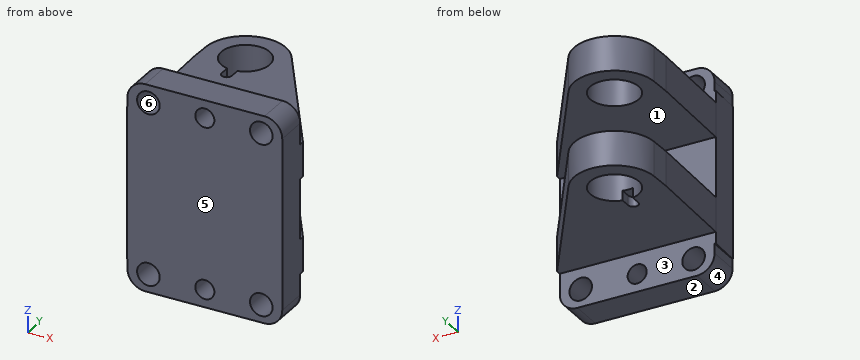
from build123d import *

# Parameters (mm, degrees)
SKETCH1_R                = 7
SKETCH1_R_2              = 5.9
BOSS_EXTRUDE1_DEPTH      = 20
BOSS_EXTRUDE2_DEPTH      = 47.15
BOSS_EXTRUDE2_DEPTH_BACK = 47.15
SKETCH3_R                = 15
BOSS_EXTRUDE3_DEPTH      = 21.4
SKETCH4_R                = 15
BOSS_EXTRUDE4_DEPTH      = 21.4
CUT_EXTRUDE1_DEPTH       = 6
CUT_EXTRUDE1_DEPTH_BACK  = 6
CUT_EXTRUDE2_DEPTH       = 6
CUT_EXTRUDE2_DEPTH_BACK  = 6


with BuildPart() as part:
    # Sketch1 → Boss-Extrude1 (new body)
    with BuildSketch(Plane(origin=(0, 0, 0), x_dir=(1, 0, 0), z_dir=(0, 1, 0))):
        with BuildLine():
            Line((-37, -64), (37, -64))
            ThreePointArc((37, -64), (44.778174593, -60.778174593), (48, -53))
            Line((48, -53), (48, 53))
            ThreePointArc((48, 53), (44.778174593, 60.778174593), (37, 64))
            Line((37, 64), (-37, 64))
            ThreePointArc((-37, 64), (-44.778174593, 60.778174593), (-48, 53))
            Line((-48, 53), (-48, -53))
            ThreePointArc((-48, -53), (-44.778174593, -60.778174593), (-37, -64))
        make_face()
        with Locations((35, 53)):
            Circle(SKETCH1_R, mode=Mode.SUBTRACT)
        with Locations((35, -53)):
            Circle(SKETCH1_R, mode=Mode.SUBTRACT)
        with Locations((0, 53)):
            Circle(SKETCH1_R_2, mode=Mode.SUBTRACT)
        with Locations((0, -53)):
            Circle(SKETCH1_R_2, mode=Mode.SUBTRACT)
        with Locations((-35, 53)):
            Circle(SKETCH1_R, mode=Mode.SUBTRACT)
        with Locations((-35, -53)):
            Circle(SKETCH1_R, mode=Mode.SUBTRACT)
    extrude(amount=BOSS_EXTRUDE1_DEPTH)

    # Sketch2 → Boss-Extrude2 (add, two sides)
    with BuildSketch(Plane.XY) as boss_extrude2_sk:
        Polygon((-48.744328002, 20), (-48.2, 0), (-43.2, 0), (-43.2, 20), align=None)
    extrude(amount=BOSS_EXTRUDE2_DEPTH)
    extrude(boss_extrude2_sk.sketch, amount=-BOSS_EXTRUDE2_DEPTH_BACK)

    # Sketch3 → Boss-Extrude3 (add)
    with BuildSketch(Plane.XY.offset(40)):
        with BuildLine():
            Line((-50.322839283, 77.998533118), (-48.2, 0))
            Line((-48.2, 0), (48, 0))
            Line((48, 0), (48, 22.55795714))
            ThreePointArc((48, 22.55795714), (47.938823082, 22.981971454), (47.760282483, 23.371399248))
            Line((47.760282483, 23.371399248), (-3.995291952, 103.55736847))
            ThreePointArc((-3.995291952, 103.55736847), (-31.752406245, 114.070833178), (-49.991433124, 90.654423708))
            Line((-49.991433124, 90.654423708), (-50.322839283, 77.998533118))
        make_face()
        with Locations((-25, 90)):
            Circle(SKETCH3_R, mode=Mode.SUBTRACT)
    extrude(amount=-BOSS_EXTRUDE3_DEPTH)

    # Sketch4 → Boss-Extrude4 (add)
    with BuildSketch(Plane.XY.offset(-40)):
        with BuildLine():
            Line((-50.322839283, 77.998533118), (-48.2, 0))
            Line((-48.2, 0), (48, 0))
            Line((48, 0), (48, 22.55795714))
            ThreePointArc((48, 22.55795714), (47.938823082, 22.981971454), (47.760282483, 23.371399248))
            Line((47.760282483, 23.371399248), (-3.995291952, 103.55736847))
            ThreePointArc((-3.995291952, 103.55736847), (-31.752406245, 114.070833178), (-49.991433124, 90.654423708))
            Line((-49.991433124, 90.654423708), (-50.322839283, 77.998533118))
        make_face()
        with Locations((-25, 90)):
            Circle(SKETCH4_R, mode=Mode.SUBTRACT)
    extrude(amount=BOSS_EXTRUDE4_DEPTH)

    # Sketch5 → Cut-Extrude1 (cut, two sides)
    with BuildSketch(Plane.XY.offset(40)) as cut_extrude1_sk:
        with BuildLine():
            Line((-21.85, 69.15), (-21.85, 90))
            Line((-21.85, 90), (-28.15, 90))
            Line((-28.15, 90), (-28.15, 69.15))
            ThreePointArc((-28.15, 69.15), (-25, 66), (-21.85, 69.15))
        make_face()
    extrude(amount=CUT_EXTRUDE1_DEPTH, mode=Mode.SUBTRACT)
    extrude(cut_extrude1_sk.sketch, amount=-CUT_EXTRUDE1_DEPTH_BACK, mode=Mode.SUBTRACT)

    # Sketch6 → Cut-Extrude2 (cut, two sides)
    with BuildSketch(Plane.XY.offset(-40)) as cut_extrude2_sk:
        with BuildLine():
            Line((-21.85, 69.15), (-21.85, 90))
            Line((-21.85, 90), (-28.15, 90))
            Line((-28.15, 90), (-28.15, 69.15))
            ThreePointArc((-28.15, 69.15), (-25, 66), (-21.85, 69.15))
        make_face()
    extrude(amount=CUT_EXTRUDE2_DEPTH, mode=Mode.SUBTRACT)
    extrude(cut_extrude2_sk.sketch, amount=-CUT_EXTRUDE2_DEPTH_BACK, mode=Mode.SUBTRACT)


solid = part.part
Build history of the part. All positions in model axes, mm. Face numbers are marked on the shaded views. A direction names the side the tool comes from. Coordinates: 2 decimals unless noted, no trailing zeros. Write each loop counter-clockwise with the first axis right and the second up, starting at its lowest first coordinate (ties: lowest second). Pieces come first, ordered by that corner, then holes.
(1) Mould opens along X. For the marked faces 4, 5 and 6 say: pulls with the +X half, pulls with the -X half, needs draft (parallel to the pull), parting line crosses it, or undercut.
(2) Drill centre lines: line 1 (Z direction, x = 0, y = 11); line 2 (X direction, y = 13, z = 53); line 3 (Z direction, x = 35, y = 5.5). Where is each one in solid material? Low to high.
(3) 3-axis set-ups, long thin cutter, end or side, ignore diameter. For the marked faces 1, 2 and 3: which of +Z, -Z, +X, -X, +Y, -Y reach the whole face in a straight line?
(4) Cut at B-B on y = 37. List the corners of the cut face in (x, z).
(5) Cut at D-D on y = 88. List the corners of the cut face in (x, z).
(6) Cut at A-A on x = -25. List the corners of the cut face in (y, z).
(7) Cut at C-C on z = -50. List the corners of the cut face in (x, y), and give its area (3 significant figures).
(8) Pin check, flat tips, straight feed: pin 1 Ø3 at (x, z) = (35, 47) entering from +Y; pin 2 Ø6 at (y, z) = (87.5, -40) entering from -X; pin 3 Ø6.5 at (y, z) = (72.5, 36.5) entering from +X; pin 4 Ø3 at (x, z) = (23, -47.5) entering from -Y. Stop position of each tip, or through.
Working result:
1. face 4: pulls with the -X half
1. face 5: needs draft
1. face 6: undercut
2. line 1: z = -64 to -58.9, -47.1 to 47.1, 58.9 to 64
2. line 2: x = -48 to -42, -28 to -5.9, 5.9 to 28, 42 to 48
2. line 3: z = -64 to -60, -46 to 46, 60 to 64
3. face 1: +X, -X, +Y
3. face 2: -Z, +X, -X, +Y, -Y
3. face 3: -Z, +X, -X, +Y
4. outline: (-49.21, -40) - (38.96, -40) - (38.96, -18.6) - (-49.21, -18.6) - close; (-49.21, 18.6) - (38.96, 18.6) - (38.96, 40) - (-49.21, 40) - close
5. outline: (-50.06, -40) - (-39.87, -40) - (-39.87, -18.6) - (-50.06, -18.6) - close; (-50.06, 18.6) - (-39.87, 18.6) - (-39.87, 40) - (-50.06, 40) - close; (-10.13, -40) - (6.05, -40) - (6.05, -18.6) - (-10.13, -18.6) - close; (-10.13, 18.6) - (6.05, 18.6) - (6.05, 40) - (-10.13, 40) - close
6. outline: (0, -64) - (20, -64) - (20, -40) - (66, -40) - (66, -34) - (75, -34) - (75, -18.6) - (20, -18.6) - (20, 18.6) - (75, 18.6) - (75, 34) - (66, 34) - (66, 40) - (20, 40) - (20, 64) - (0, 64) - close; (105, -40) - (115, -40) - (115, -18.6) - (105, -18.6) - close; (105, 18.6) - (115, 18.6) - (115, 40) - (105, 40) - close
7. outline: (-48, 0) - (-41.32, 0) - (-41.32, 20) - (-48, 20) - close; (-28.68, 0) - (-5.08, 0) - (-5.08, 20) - (-28.68, 20) - close; (5.08, 0) - (28.68, 0) - (28.68, 20) - (5.08, 20) - close; (41.32, 0) - (48, 0) - (48, 20) - (41.32, 20) - close
7. area: 1,210 mm2
8. pin 1: stops at y = 20
8. pin 2: stops at x = -50.15
8. pin 3: stops at x = 18.15
8. pin 4: stops at y = 0
